Build history of the part. All positions in model axes, mm. Round coordinates to 2 decimals unless told otherwise and drop trailing zeros. Order: outer loops, then holes, each group sorted by start corner. A loop starts at its lowest first (then second) coordinate and runs counter-clockwise, first axis right, second up. Notation, with made-up numbers: (81.25, 6.25) -> (131.25, 6.25) arc R26 ccw to (131.25, 35.25) -> close; hole circle Ø5 at (68, 65). An arc over 180 degrees is marked (long way). Answer as a JSON object with one key per item and string values.
from build123d import *

# Parameters (mm, degrees)
F1_DEPTH = 3.175


with BuildPart() as f1:
    # F0 (on Top) → F1 (new body)
    with BuildSketch(Plane.XY):
        Polygon((24.269844, -44.48778), (24.269844, -64.80778), (30.619844, -64.80778), (30.619844, -58.45778), (43.319844, -58.45778), (43.319844, -64.80778), (62.369844, -64.80778), (62.369844, -58.45778), (81.419844, -58.45778), (81.419844, -64.80778), (100.469844, -64.80778), (100.469844, -58.45778), (119.519844, -58.45778), (119.519844, -64.80778), (138.569844, -64.80778), (138.569844, -58.45778), (157.619844, -58.45778), (157.619844, -64.80778), (170.319844, -64.80778), (183.019844, -64.80778), (183.019844, -58.45778), (202.069844, -58.45778), (202.069844, -64.80778), (221.119844, -64.80778), (221.119844, -58.45778), (240.169844, -58.45778), (240.169844, -64.80778), (259.219844, -64.80778), (259.219844, -58.45778), (278.269844, -58.45778), (278.269844, -64.80778), (297.319844, -64.80778), (297.319844, -58.45778), (310.019844, -58.45778), (310.019844, -64.80778), (316.369844, -64.80778), (316.369844, -44.48778), (322.719844, -44.48778), (322.719844, -24.16778), (316.369844, -24.16778), (316.369844, -3.84778), (322.719844, -3.84778), (322.719844, 16.47222), (316.369844, 16.47222), (316.369844, 30.44222), (297.319844, 30.44222), (297.319844, 36.79222), (278.269844, 36.79222), (278.269844, 30.44222), (259.219844, 30.44222), (259.219844, 36.79222), (240.169844, 36.79222), (240.169844, 30.44222), (221.119844, 30.44222), (221.119844, 36.79222), (202.069844, 36.79222), (202.069844, 30.44222), (183.019844, 30.44222), (183.019844, 36.79222), (170.319844, 36.79222), (157.619844, 36.79222), (157.619844, 30.44222), (138.569844, 30.44222), (138.569844, 36.79222), (119.519844, 36.79222), (119.519844, 30.44222), (100.469844, 30.44222), (100.469844, 36.79222), (81.419844, 36.79222), (81.419844, 30.44222), (62.369844, 30.44222), (62.369844, 36.79222), (43.319844, 36.79222), (43.319844, 30.44222), (24.269844, 30.44222), (24.269844, 16.47222), (17.919844, 16.47222), (17.919844, -3.84778), (24.269844, -3.84778), (24.269844, -24.16778), (17.919844, -24.16778), (17.919844, -44.48778), align=None)
    extrude(amount=F1_DEPTH)


solid = f1.part
1) Flat gauge pins, fed straight in: pin 1 Ø1 at (x, z) = (309.5, 1) entering from +Y; pin 2 Ø10 at (x, y) = (164.5, -26) entering from -Z; pin 3 Ø1 at (y, z) = (33.5, 1) entering from +X; pin 4 Ø1 at (x, z) = (20.5, 1.5) entering from +Y. Where does each tip first touch, or does it go through?
Checked values:
{"pin 1": "stops at y = 30.44", "pin 2": "stops at z = 0", "pin 3": "stops at x = 297.32", "pin 4": "stops at y = 16.47"}
2) Cut at A-A, the plane y = 26. Give the cut face in (x, z) (3 decimals).
Checked values:
{"outline": "(24.27, 0) -> (316.37, 0) -> (316.37, 3.175) -> (24.27, 3.175) -> close"}
3) Cut at B-B, the plane x = 192. Give the cut face in (y, z) (3 decimals).
Checked values:
{"outline": "(-58.458, 0) -> (30.442, 0) -> (30.442, 3.175) -> (-58.458, 3.175) -> close"}
4) Probe L1, parallel to X at y = -53, z = 2.8; L2, parallel to Y at x = 146, z = 1.05. List the from-to ranges inside material, lowest first. Write a range as from..to.
Checked values:
{"L1": "x = 24.27..316.37", "L2": "y = -58.46..30.44"}
